Geometry: final body of the model. Coordinates: model frame, mm. Face numbers are marked on the shaded views. Coordinates: 2 decimals unless noted, no trailing zeros. Write each loop counter-clockwise with the first axis right and the second up, starting at its lowest first coordinate (ties: lowest second). Pieces come first, ordered by that corner, then holes. Notation, with made-up numbers: M -15.5,-19 L 28.5,-19 A15 cw 28.5,-3 Z; hole C 47,64 d1. An arc over 180 degrees is marked long. Write item = value, one per line. Start each with the question number.
Item 1: Pull-direction query (Z, two-part tool) for the marked faces 1, 2, 3 and 4; classes: +Z half, -Z half, draft (parallel to the pull), parting line (faces both ways), or undercut.
Item 2: Section D-D on z = -13. Output: boundary loops of the cut face in (x, y), plus the area to 3 significant figures.
Item 3: Ray query, L1, parallel to X at y = 0.95, z = -10.15 (3 decimals); L2, parallel to X at y = 2.9, z = -10.15 (3 decimals); L3, parallel to X at y = 2.8, z = -10.15 (3 decimals). Return the intervals inside material, ascending. Write a range as [from, to].
Item 4: First-contact query: pin 1 Ø1.9 at (x, z) = (14, -10.15) entering from +Y; pin 2 Ø2 at (x, y) = (8.5, 1) entering from +Z; pin 3 Ø1.5 at (y, z) = (3.5, -3.5) entering from -X. Flat tips, straight axial feed; report the tip coordinate or a pass-through.
Item 5: Section A-A on y = 1.75. Output: boundary loops of the cut face in (x, z) (3 decimals), plus the area to 3 significant figures.
Item 6: Section C-C on y = 3.65. Output: boundary loops of the cut face in (x, z) (3 decimals), plus the area to 3 significant figures.
Item 7: Section B-B on x = 14. Output: boundary loops of the cut face in (y, z) (3 decimals).
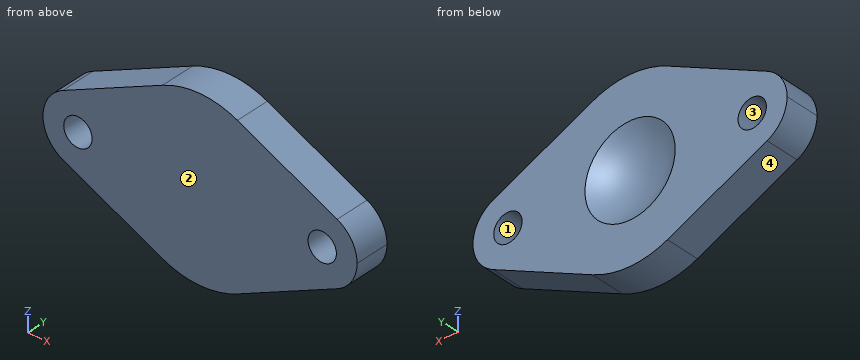
from build123d import *

# Parameters (mm, degrees)
CROQUIS1_W              = 36
CROQUIS1_H              = 20.3
CROQUIS1_R              = 1.625
SALIENTE_EXTRUIR1_DEPTH = 4
CORTAR_EXTRUIR2_DEPTH   = 28.424259334


with BuildPart() as part:
    # Croquis1 → Saliente-Extruir1 (new body)
    with BuildSketch(Plane(origin=(0, 0, 0), x_dir=(1, 0, 0), z_dir=(0, 1, 0))):
        with Locations((0, 10.15)):
            Rectangle(CROQUIS1_W, CROQUIS1_H)
        with Locations(Location((-14, 10.15, 0), (0, 0, 270))):
            Circle(CROQUIS1_R, mode=Mode.SUBTRACT)
        with Locations(Location((14, 10.15, 0), (0, 0, 90))):
            Circle(CROQUIS1_R, mode=Mode.SUBTRACT)
    extrude(amount=SALIENTE_EXTRUIR1_DEPTH)

    # Croquis2 → Cortar-Revolución1 (revolve, cut)
    with BuildSketch(Plane.XY.offset(-10.15)):
        with BuildLine():
            Line((0, 18.45), (0, 2.15))
            ThreePointArc((0, 2.15), (-8.15, 10.3), (0, 18.45))
        make_face()
    revolve(axis=Axis((0, -1000, -10.15), (0, 1, 0)), mode=Mode.SUBTRACT)

    # Croquis3 → Cortar-Extruir2 (cut, through all)
    with BuildSketch(Plane(origin=(0, 4, 0), x_dir=(1, 0, 0), z_dir=(0, 1, 0))):
        with BuildLine():
            ThreePointArc((-18, 10.15), (-17.380616997, 12.288089971), (-15.714285638, 13.764031648))
            Line((-15.714285638, 13.764031648), (-4.285714096, 19.185078825))
            ThreePointArc((-4.285714096, 19.185078825), (1.05e-07, 20.149999706), (4.285714286, 19.185078735))
            Line((4.285714286, 19.185078735), (15.714285714, 13.764031612))
            ThreePointArc((15.714285714, 13.764031612), (17.380617007, 12.288089954), (18, 10.150000044))
            Line((18, 10.150000044), (18, 20.3))
            Line((18, 20.3), (-18, 20.3))
            Line((-18, 20.3), (-18, 10.15))
        make_face()
        with BuildLine():
            ThreePointArc((-15.714285714, 6.535968388), (-17.380617019, 8.011910065), (-18, 10.15))
            Line((-18, 10.15), (-18, -5.88e-07))
            Line((-18, -5.88e-07), (18, -5.88e-07))
            Line((18, -5.88e-07), (18, 10.150000044))
            ThreePointArc((18, 10.150000044), (17.380617031, 8.011910083), (15.714285714, 6.535968388))
            Line((15.714285714, 6.535968388), (4.285714286, 1.114920677))
            ThreePointArc((4.285714286, 1.114920677), (0, 0.149999706), (-4.285714286, 1.114920677))
            Line((-4.285714286, 1.114920677), (-15.714285714, 6.535968388))
        make_face()
    extrude(amount=-CORTAR_EXTRUIR2_DEPTH, mode=Mode.SUBTRACT)


solid = part.part
Responses:
q1.face_1 = undercut
q1.face_2 = draft
q1.face_3 = undercut
q1.face_4 = -Z half
q2.outline = M -16.81,0 L 16.81,0 L 16.81,4 L 4.31,4 A7.64 cw -4.31,4 L -16.81,4 Z
q2.area = 127 mm²
q3.L1 = [-18, -15.625], [-12.375, 12.375], [15.625, 18]
q3.L2 = [-18, -15.625], [-12.375, -3.415], [3.415, 12.375], [15.625, 18]
q3.L3 = [-18, -15.625], [-12.375, -3.189], [3.189, 12.375], [15.625, 18]
q4.pin_1 = through
q4.pin_2 = -2.64
q4.pin_3 = -10.9
q5.outline = M -15.714,-13.764 L -4.286,-19.185 A10 ccw 4.286,-19.185 L 15.714,-13.764 A4 ccw 15.714,-6.536 L 4.286,-1.115 A10 ccw -4.286,-1.115 L -15.714,-6.536 A4 ccw Z; hole C -14,-10.15 d3.25; hole C 14,-10.15 d3.25
q5.area = 462 mm²
q6.outline = M -15.714,-13.764 L -4.286,-19.185 A10 ccw 4.286,-19.185 L 15.714,-13.764 A4 ccw 15.714,-6.536 L 4.286,-1.115 A10 ccw -4.286,-1.115 L -15.714,-6.536 A4 ccw Z; hole C -14,-10.15 d3.25; hole C 0,-10.15 d9.423; hole C 14,-10.15 d3.25
q6.area = 393 mm²
q7.outline = M 0,-14.577 L 4,-14.577 L 4,-11.775 L 0,-11.775 Z; M 0,-8.525 L 4,-8.525 L 4,-5.723 L 0,-5.723 Z
